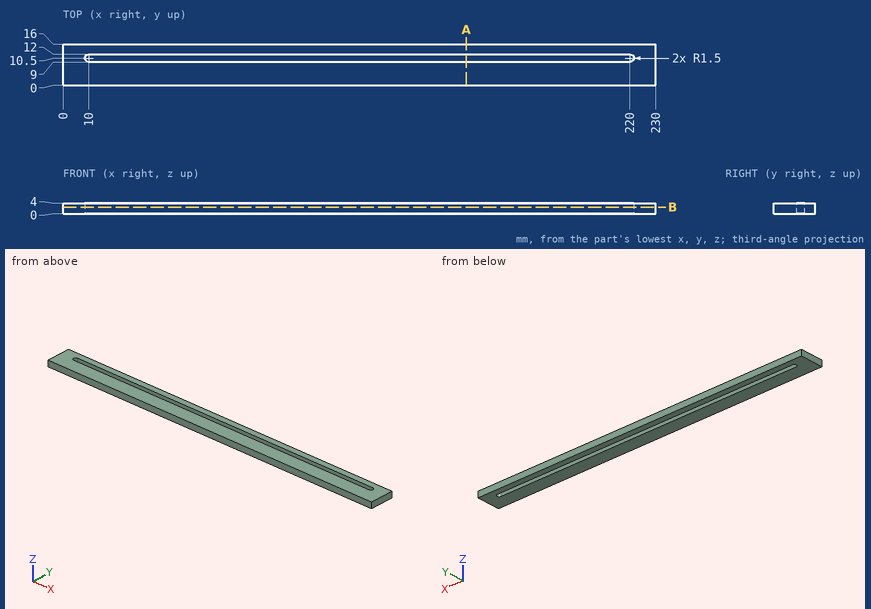
The figure shows three views and two pictorial views of one solid part (mm, origin at its lowest corner). Answer the questions. Round coordinates to 2 decimals unless told otherwise and drop trailing zeros. Loops run counter-clockwise (first coordinate to the right, second up) from the corner with the lowest first, then second, coordinate; pieces in that order, holes last. Notation, with made-up numbers: M 25.5,71.25 L 54.5,71.25 A21 cw 54.5,96.25 Z; hole C -20,-3 d4. An arc over 180 degrees is marked long. Write each question's results on one line, items separated by ' | '. Start each with the question number.
1) Find section B-B on z = 2.5. Write down the section's boundary in (x, y).
2) Find section A-A on x = 156.5. Write down the section's boundary in (y, z).
3) Straight lines are drawn through the part: probe 1 along Y at (x, z) = (20, 3); probe 2 along X at (y, z) = (11, 0.7); probe 3 along X at (y, z) = (11.5, 2.25). For each, find the intervals that lie inside material, in ascending order.
Final values:
1) outline: M 0,0 L 230,0 L 230,16 L 0,16 Z; hole M 10,9 L 220,9 A1.5 ccw 220,12 L 10,12 A1.5 ccw Z
2) outline: M 0,0 L 9,0 L 9,4 L 0,4 Z; M 12,0 L 16,0 L 16,4 L 12,4 Z
3) probe 1: 0 to 9, 12 to 16 | probe 2: 0 to 8.59, 221.41 to 230 | probe 3: 0 to 8.88, 221.12 to 230
